from build123d import *

# Parameters (mm, degrees)
F1_DEPTH = 1.5875
F2_R     = 19.04999
F3_R     = 6.35
F4_R     = 15.875
F5_DEPTH = 25.4
F6_W     = 63.5
F6_H     = 3.175
F7_DEPTH = 25.4
F8_R     = 1.58749


# Not quite as in the source:
# - a fillet or chamfer is up to 0.001 mm smaller than in the source, because OpenCascade refuses the exact size


with BuildPart() as f1:
    # F0 (on Right) → F1 (new body)
    with BuildSketch(Plane.YZ):
        Polygon((-63.1363113923, 43.5325428513), (-101.2363113923, 43.5325428513), (-101.2363113923, 5.4325428513), (57.5136886077, 5.4325428513), (57.5136886077, -13.6174602094), (63.8636886077, -13.6174602094), (63.8636886077, 18.1325428513), (-63.1363113923, 18.1325428513), align=None)
    extrude(amount=F1_DEPTH)

    # F2 (radius 19.05 in the source; OpenCascade refuses exactly that, so slightly less here)
    f2_edges = [f1.edges().sort_by_distance(p)[0] for p in [
        (0.79375, -63.136311, 43.532543),
        (0.79375, -101.236311, 43.532543),
        (0.79375, -101.236311, 5.432543),
    ]]
    fillet(f2_edges, radius=F2_R)

    # F3
    f3_edges = [f1.edges().sort_by_distance(p)[0] for p in [
        (0.79375, -63.136311, 18.132543),
    ]]
    fillet(f3_edges, radius=F3_R)

    # F4 (on face) → F5 (cut)
    with BuildSketch(Plane.YZ.offset(1.5875)):
        with Locations((-82.1863113923, 24.4825428513)):
            Circle(F4_R)
    extrude(amount=-F5_DEPTH, mode=Mode.SUBTRACT)

    # F6 (on face) → F7 (cut)
    with BuildSketch(Plane.YZ.offset(1.5875)):
        with Locations((19.4136886077, 11.7825428513)):
            Rectangle(F6_W, F6_H)
    extrude(amount=-F7_DEPTH, mode=Mode.SUBTRACT)

    # F8 (radius 1.5875 in the source; OpenCascade refuses exactly that, so slightly less here)
    f8_edges = [f1.edges().sort_by_distance(p)[0] for p in [
        (0.79375, -12.336311, 13.370043),
        (0.79375, -12.336311, 10.195043),
        (0.79375, 51.163689, 10.195043),
        (0.79375, 51.163689, 13.370043),
    ]]
    fillet(f8_edges, radius=F8_R)


solid = f1.part
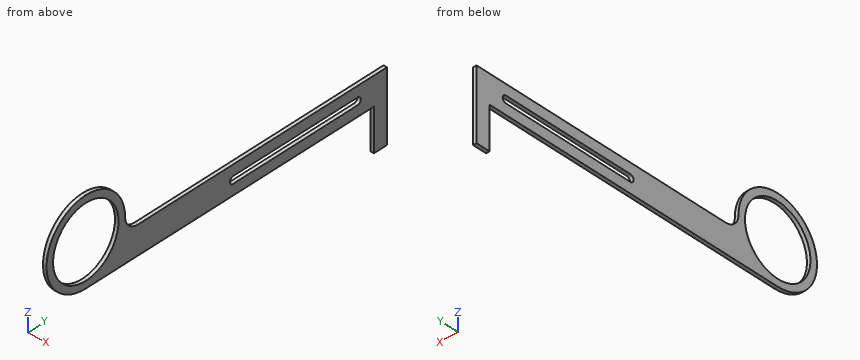
Here's how the part is built. I have some questions about the finished solid (model axes, mm). Coordinates: 2 decimals unless noted, no trailing zeros. Order: outer loops, then holes, each group sorted by start corner. A loop starts at its lowest first (then second) coordinate and runs counter-clockwise, first axis right, second up. Notation, with made-up numbers: M 77,-22.5 L 109,-22.5 A23 cw 109,11.5 Z; hole C 52.5,32 d7. An arc over 180 degrees is marked long. Answer as CSV lines item,"result". Start each with the question number.
1. I want a section at C-C, the plane z = 38. Write out the boundary of the cut face in (x, y).
2. I need wall thicknesses on line 1 (Z direction, x = 1, y = -10.5); line 2 (Y direction, x = 1.35, z = 12); line 3 (Z direction, x = 0.3, y = -57). Which ranges of each line are inside material? Lowest first, please. Write a range as [from, to].
3. I want a section at B-B, the plane x = 1.2. Count the separate pieces of the cut face and the enclosed holes in it, and give its area (3 significant figures).
4. I want a section at A-A, the plane y = 0. Write out the boundary of the cut face in (x, z).
5. I want a section at D-D, the plane z = -3. Write out the boundary of the cut face in (x, y).
6. For pin 1 (0.5 mm diameter, centred on x = 0.5, y = 23.5, fed in from -Z); pin 2 (0.8 mm diameter, centred on x = 1, y = -1, fed in from +Z); pin 3 (0.5 mm diameter, centred on x = 0.5, z = 0, fed in from -Y), each with a flat end and sliding along its axis, tell me the tip position at first contact or that it passes through.
Recorded:
1,outline,"M 0,-95.61 L 1.59,-95.61 L 1.59,-90.51 L 0,-90.51 Z; M 0,-73.86 L 1.59,-73.86 L 1.59,-68.76 L 0,-68.76 Z"
2,line 1,"z = [5.43, 10.2], [13.37, 18.13]"
2,line 2,"y = [-96.58, -91.99], [-72.38, -12.32], [51.15, 63.86]"
2,line 3,"z = [5.43, 18.14]"
3,separate pieces,"1"
3,enclosed holes,"2"
3,area,"1,970 mm2"
4,outline,"M 0,5.43 L 1.59,5.43 L 1.59,10.2 L 0,10.2 Z; M 0,13.37 L 1.59,13.37 L 1.59,18.13 L 0,18.13 Z"
5,outline,"M 0,57.51 L 1.59,57.51 L 1.59,63.86 L 0,63.86 Z"
6,pin 1,"stops at z = 5.43"
6,pin 2,"stops at z = 18.13"
6,pin 3,"stops at y = 57.51"
